Model file for the job. Use its own axes, mm. A direction names the side the tool comes from. Give positions to 0.01 mm unless a question says otherwise; leave off trailing zeros. Loops run counter-clockwise (first coordinate to the right, second up) from the corner with the lowest first, then second, coordinate; pieces in that order, holes last. Notation, with made-up numbers: (31, -12.75) - (79, -12.75) arc R18 ccw to (79, -7.75) - close; hole circle Ø3 at (71.25, -38.5). An arc over 180 degrees is marked (long way). Use a Markdown table: item, result.
from build123d import *

# Parameters (mm, degrees)
CYLINDER007_R     = 3
CYLINDER007_DEPTH = 5
CYLINDER008_R     = 3
CYLINDER008_DEPTH = 5
CYLINDER009_R     = 3
CYLINDER009_DEPTH = 5
CYLINDER006_R     = 3
CYLINDER006_DEPTH = 5
CYLINDER005_R     = 1.5
CYLINDER005_DEPTH = 25
CYLINDER004_R     = 1.5
CYLINDER004_DEPTH = 25
CYLINDER003_R     = 1.5
CYLINDER003_DEPTH = 25
CYLINDER002_R     = 1.5
CYLINDER002_DEPTH = 25
CYLINDER001_R     = 10.25
CYLINDER001_DEPTH = 25
CYLINDER_R        = 21.25
CYLINDER_DEPTH    = 25


with BuildPart() as zylinder007:
    # Cylinder007 → Cylinder007 (new body)
    with BuildSketch(Plane(origin=(0, 15, 0), x_dir=(1, 0, 0), z_dir=(0, 0, 1))):
        Circle(CYLINDER007_R)
    extrude(amount=CYLINDER007_DEPTH)


with BuildPart() as zylinder008:
    # Cylinder008 → Cylinder008 (new body)
    with BuildSketch(Plane(origin=(-15, 0, 0), x_dir=(1, 0, 0), z_dir=(0, 0, 1))):
        Circle(CYLINDER008_R)
    extrude(amount=CYLINDER008_DEPTH)


with BuildPart() as zylinder009:
    # Cylinder009 → Cylinder009 (new body)
    with BuildSketch(Plane(origin=(0, -15, 0), x_dir=(1, 0, 0), z_dir=(0, 0, 1))):
        Circle(CYLINDER009_R)
    extrude(amount=CYLINDER009_DEPTH)


with BuildPart() as zylinder006:
    # Cylinder006 → Cylinder006 (new body)
    with BuildSketch(Plane(origin=(15, 0, 0), x_dir=(1, 0, 0), z_dir=(0, 0, 1))):
        Circle(CYLINDER006_R)
    extrude(amount=CYLINDER006_DEPTH)


with BuildPart() as zylinder005:
    # Cylinder005 → Cylinder005 (new body)
    with BuildSketch(Plane(origin=(0, -15, 0), x_dir=(1, 0, 0), z_dir=(0, 0, 1))):
        Circle(CYLINDER005_R)
    extrude(amount=CYLINDER005_DEPTH)


with BuildPart() as zylinder004:
    # Cylinder004 → Cylinder004 (new body)
    with BuildSketch(Plane(origin=(-15, 0, 0), x_dir=(1, 0, 0), z_dir=(0, 0, 1))):
        Circle(CYLINDER004_R)
    extrude(amount=CYLINDER004_DEPTH)


with BuildPart() as zylinder003:
    # Cylinder003 → Cylinder003 (new body)
    with BuildSketch(Plane(origin=(0, 15, 0), x_dir=(1, 0, 0), z_dir=(0, 0, 1))):
        Circle(CYLINDER003_R)
    extrude(amount=CYLINDER003_DEPTH)


with BuildPart() as zylinder002:
    # Cylinder002 → Cylinder002 (new body)
    with BuildSketch(Plane(origin=(15, 0, 0), x_dir=(1, 0, 0), z_dir=(0, 0, 1))):
        Circle(CYLINDER002_R)
    extrude(amount=CYLINDER002_DEPTH)


with BuildPart() as zylinder001:
    # Cylinder001 → Cylinder001 (new body)
    with BuildSketch(Plane.XY):
        Circle(CYLINDER001_R)
    extrude(amount=CYLINDER001_DEPTH)


with BuildPart() as cut008:
    # Cylinder → Cylinder (new body)
    with BuildSketch(Plane.XY):
        Circle(CYLINDER_R)
    extrude(amount=CYLINDER_DEPTH)

    # Cut: cut Zylinder001
    add(zylinder001.part, mode=Mode.SUBTRACT)

    # Cut001: cut Zylinder002
    add(zylinder002.part, mode=Mode.SUBTRACT)

    # Cut002: cut Zylinder003
    add(zylinder003.part, mode=Mode.SUBTRACT)

    # Cut003: cut Zylinder004
    add(zylinder004.part, mode=Mode.SUBTRACT)

    # Cut004: cut Zylinder005
    add(zylinder005.part, mode=Mode.SUBTRACT)

    # Cut005: cut Zylinder006
    add(zylinder006.part, mode=Mode.SUBTRACT)

    # Cut006: cut Zylinder009
    add(zylinder009.part, mode=Mode.SUBTRACT)

    # Cut007: cut Zylinder008
    add(zylinder008.part, mode=Mode.SUBTRACT)

    # Cut008: cut Zylinder007
    add(zylinder007.part, mode=Mode.SUBTRACT)


solid = cut008.part
(1) Slice it at C-C, the plane y = -15. Write the cut outline in (x, z), plus the area to 3 significant figures.
Computed:
| item | result |
|---|---|
| outline | (-15.05, 0) - (-3, 0) - (-3, 5) - (-1.5, 5) - (-1.5, 25) - (-15.05, 25) - close; (1.5, 5) - (3, 5) - (3, 0) - (15.05, 0) - (15.05, 25) - (1.5, 25) - close |
| area | 663 mm² |
(2) Slice it at B-B, the plane z = 1.5. Write the cut outline in (x, y).
Computed:
| item | result |
|---|---|
| outline | circle Ø42.5 at (0, 0); hole circle Ø6 at (-15, 0); hole circle Ø20.5 at (0, 0); hole circle Ø6 at (0, -15); hole circle Ø6 at (0, 15); hole circle Ø6 at (15, 0) |
(3) Drill centre lines: probe 1 along Y at (x, z) = (0, 7.5); probe 2 along Y at (x, z) = (0, 3.9); probe 3 along X at (y, z) = (-15, 14.75). Where is each one in solid material? Low to high. Write a range as [from, to].
Computed:
| item | result |
|---|---|
| probe 1 | [-21.25, -16.5], [-13.5, -10.25], [10.25, 13.5], [16.5, 21.25] |
| probe 2 | [-21.25, -18], [-12, -10.25], [10.25, 12], [18, 21.25] |
| probe 3 | [-15.05, -1.5], [1.5, 15.05] |
(4) 3-axis set-ups, long thin cutter, end or side, ignore diameter. For faces 4 (the flat face through (1.3, 13.7, 5)), 5 (the flat face through (9.15, 5.02, 0)): which of +Z, -Z, +X, -X, +Y, -Y reach the whole face in a straight line?
Computed:
| item | result |
|---|---|
| face 4 | -Z |
| face 5 | -Z, +X, -X, +Y, -Y |
(5) Mould opens along Y. For faces 1 (the cylindrical face through (-0.65, 12.07, 2.46)), 2 (the flat face through (9.15, 5.02, 25)), 3 (the cylindrical face through (-16.863, -12.93, 12.325)) say: pulls with the +Y half, pulls with the -Y half, needs draft (parallel to the pull), parting line crosses it, or undercut.
Computed:
| item | result |
|---|---|
| face 1 | undercut |
| face 2 | needs draft |
| face 3 | parting line crosses it |
(6) Slice it at A-A, the plane x = 0. Write the cut outline in (y, z).
Computed:
| item | result |
|---|---|
| outline | (-21.25, 0) - (-18, 0) - (-18, 5) - (-16.5, 5) - (-16.5, 25) - (-21.25, 25) - close; (-13.5, 5) - (-12, 5) - (-12, 0) - (-10.25, 0) - (-10.25, 25) - (-13.5, 25) - close; (10.25, 0) - (12, 0) - (12, 5) - (13.5, 5) - (13.5, 25) - (10.25, 25) - close; (16.5, 5) - (18, 5) - (18, 0) - (21.25, 0) - (21.25, 25) - (16.5, 25) - close |
(7) Slice it at D-D, the plane x = -5. Write the cut outline in (y, z), plus the area to 3 significant figures.
Computed:
| item | result |
|---|---|
| outline | (-20.65, 0) - (-8.95, 0) - (-8.95, 25) - (-20.65, 25) - close; (8.95, 0) - (20.65, 0) - (20.65, 25) - (8.95, 25) - close |
| area | 585 mm² |
(8) Pin check, flat tips, straight feed: P1, Ø12, axis at x = -5, z = 12.5, coming from the +Y side; P2, Ø1, axis at x = 8, y = 4, coming from the -Z side; P3, Ø3, axis at x = 15.5, y = 0, coming from the -Z side; P4, Ø1.5, axis at x = 11.5, z = 17.5, coming from the -Y side. Stop position of each tip, or through.
Computed:
| item | result |
|---|---|
| P1 | y = 21.25 |
| P2 | through |
| P3 | z = 5 |
| P4 | y = -18.33 |
